Verification items for the finished model (mm, model axes). Round coordinates to 2 decimals unless told otherwise and drop trailing zeros. Write each loop counter-clockwise with the first axis right and the second up, starting at its lowest first coordinate (ties: lowest second). Pieces come first, ordered by that corner, then holes. Notation, with made-up numbers: (14.25, 61.5) -> (40.25, 61.5) arc R20 cw to (40.25, 92.5) -> close; hole circle Ø8 at (80.25, 21.5). An arc over 180 degrees is marked (long way). Answer as a JSON object with one key per item and string values. Group by question number.
(1) Sectioned sample at A-A on x = 32.8. Record the cut outline in (y, z) (3 decimals).
(2) Sectioned sample at B-B on z = 55. Record the cut outline in (x, y) (3 decimals).
(3) Sectioned sample at D-D on z = 32. Record the cut outline in (x, y), and give its area (3 significant figures).
(4) Draft check along Z on faces 1 (the face through (32, 0, 42)), 2 (the face through (30.74, 0.91, 64.3)). Enter one of: released by +Z, released by -Z, zero draft, split by the parting line, or undercut.
(5) Sectioned sample at C-C on y = 0.8. Record the cut outline in (x, z) (3 decimals), and give its area (3 significant figures).
(6) Gauge pin test, flat ends, axial feed: pin 1 Ø1 at (y, z) = (1.5, 21) entering from +X; pin 2 Ø11.5 at (x, z) = (32.8, 55) entering from +Y. Record the tip position at first contact, or that the pin passes through.
(7) Scan lines: L1, parallel to Z at x = 32.5, y = 1.15; L2, parallel to Z at x = 25, y = 0.6; L3, parallel to X at y = 1.25, z = 55 (3 decimals). Record each from-to range of solid material in increasing order. Write a range as from..to.
```python
from build123d import *

# Parameters (mm, degrees)
BOSS_EXTRUDE1_DEPTH = 110
SKETCH2_R           = 9.525
CUT_EXTRUDE1_DEPTH  = 2.8


with BuildPart() as part:
    # Sketch1 → Boss-Extrude1 (new body)
    with BuildSketch(Plane.XY):
        Polygon((0, 0), (65.6, 0), (63.8, 1.8), (1.8, 1.8), align=None)
    extrude(amount=BOSS_EXTRUDE1_DEPTH)

    # Sketch2 → Cut-Extrude1 (cut, through all)
    with BuildSketch(Plane(origin=(0, 1.8, 0), x_dir=(1, 0, 0), z_dir=(0, 1, 0))):
        with Locations((32.8, -55)):
            Circle(SKETCH2_R)
    extrude(amount=-CUT_EXTRUDE1_DEPTH, mode=Mode.SUBTRACT)


solid = part.part
```
Computed values:
{
 "1": {"outline": "(0, 0) -> (1.8, 0) -> (1.8, 45.475) -> (0, 45.475) -> close; (0, 64.525) -> (1.8, 64.525) -> (1.8, 110) -> (0, 110) -> close"},
 "2": {"outline": "(0, 0) -> (23.275, 0) -> (23.275, 1.8) -> (1.8, 1.8) -> close; (42.325, 0) -> (65.6, 0) -> (63.8, 1.8) -> (42.325, 1.8) -> close"},
 "3": {"outline": "(0, 0) -> (65.6, 0) -> (63.8, 1.8) -> (1.8, 1.8) -> close", "area": "115 mm2"},
 "4": {"face 1": "zero draft", "face 2": "undercut"},
 "5": {"outline": "(0.8, 0) -> (64.8, 0) -> (64.8, 110) -> (0.8, 110) -> close; hole circle Ø19.05 at (32.8, 55)", "area": "6,750 mm2"},
 "6": {"pin 1": "x = 64.6", "pin 2": "through"},
 "7": {"L1": "0..45.48, 64.52..110", "L2": "0..49.53, 60.47..110", "L3": "1.25..23.275, 42.325..64.35"}
}
